Solid Edge part; units mm, degrees
sketch "Sketch1" plane through (0, 0, 0) normal (0, 0, 1) x (1, 0, 0)
  circle A0 centre (0, 0) radius 3.3
extrude "Protrusion1" add sketch "Sketch1" along normal blind 4.8
sketch "Sketch2" plane through (0, 0, 4.8) normal (0, 0, 1) x (1, 0, 0)
  circle A0 centre (0, 0) radius 2.25
extrude "nail_base" cut sketch "Sketch2" against normal blind 0.8
sketch "Sketch3" plane through (0, 0, 4) normal (0, 0, 1) x (1, 0, 0)
  circle A0 centre (0, 0) radius 1.4
extrude "Cutout1" cut sketch "Sketch3" against normal through all
sketch "Sketch4" plane through (0, 0, 0) normal (0, 0, -1) x (0, 1, 0)
  circle A0 centre (0, 0) radius 2.2
extrude "servo_mounting" cut sketch "Sketch4" against normal blind 2.8
sketch "Sketch5" plane through (0, 0, 2.4) normal (0, 0, -1) x (1, 0, 0)
  line L0 (-3.2891, 0.268) -> (-1.95, 16.7)
  arc A0 (-1.95, 16.7) -> (1.95, 16.7) centre (0, 16.1825) cw
  line L1 (3.2891, 0.268) -> (1.95, 16.7)
  arc A1 (-3.2891, 0.268) -> (3.2891, 0.268) centre (0, 0) cw
extrude "connector" add sketch "Sketch5" against normal blind 2
sketch "Sketch6" plane through (0, 0, 0) normal (0, 0, 1) x (1, 0, 0)
  circle A0 centre (0, -4.9) radius 0.6
  circle A1 centre (0, -6.8333) radius 0.6
  circle A2 centre (0, -8.7667) radius 0.6
  circle A3 centre (0, -10.7) radius 0.6
  circle A4 centre (0, -12.6333) radius 0.6
  circle A5 centre (0, -14.5667) radius 0.6
  circle A6 centre (0, -16.5) radius 0.6
extrude "Cutout2" cut sketch "Sketch6" along normal through all
The listing builds one solid part. Answer for the finished solid, in the listing's coordinates (mm). A direction names the side the tool comes from. Give positions to 0.01 mm unless a question says otherwise; leave off trailing zeros. Order: outer loops, then holes, each group sorted by start corner. A loop starts at its lowest first (then second) coordinate and runs counter-clockwise, first axis right, second up.
Item 1: The part is cut by section A-A, the plane y = 0. Give the vertices of the cut face in (x, z), and give its area (3 significant figures).
From the geometry:
outline: (-3.3, 0) - (-2.2, 0) - (-2.2, 2.8) - (-1.4, 2.8) - (-1.4, 4) - (-2.25, 4) - (-2.25, 4.8) - (-3.3, 4.8) - close; (1.4, 2.8) - (2.2, 2.8) - (2.2, 0) - (3.3, 0) - (3.3, 4.8) - (2.25, 4.8) - (2.25, 4) - (1.4, 4) - close
area: 12.4 mm2
Item 2: For a pull along X with two mould halves and no side action, classify faces 4 (the face through (1.4, -2.2, 4.8)), 5 (the face through (0.277, -14.034, 3.386)), 6 (the face through (-2.63, -8.37, 3.39)) as pulls with the +X half, pulls with the -X half, needs draft (parallel to the pull), parting line crosses it, or undercut.
From the geometry:
face 4: needs draft
face 5: undercut
face 6: pulls with the -X half
Item 3: The part is cut by section D-D, the plane y = -16.5. Give the vertices of the cut face in (x, z), and give its area (3 significant figures).
From the geometry:
outline: (-1.97, 2.4) - (-0.6, 2.4) - (-0.6, 4.4) - (-1.97, 4.4) - close; (0.6, 2.4) - (1.97, 2.4) - (1.97, 4.4) - (0.6, 4.4) - close
area: 5.47 mm2
Item 4: Which of the six approach directions +Z, -Z, +X, -X, +Y, -Y give full straight-line access (tool end or side, diameter ignored) to faces 1 (the face through (-0.078, -17.095, 3.386)), 2 (the face through (-0.29, 2.23, 4.41)), 3 (the face through (0.66, 2.1, 1.38))?
From the geometry:
face 1: +Z, -Z
face 2: +Z
face 3: -Z
Item 5: Find the intervals of material crossed by probe 1 along X at (y, z) = (-16.5, 3.8); probe 2 along Z at (x, y) = (1, -6); probe 3 along Y at (x, z) = (1, 1.25), in increasing order.
From the geometry:
probe 1: x = -1.97 to -0.6, 0.6 to 1.97
probe 2: z = 2.4 to 4.4
probe 3: y = -3.14 to -1.96, 1.96 to 3.14
Item 6: Given pin 1 Ø1.9 at (x, y) = (0, -6.83) entering from +Z; pin 2 Ø3 at (x, y) = (-2.5, -9.5) entering from -Z; pin 3 Ø1.3 at (x, y) = (0, 1) entering from +Z; pin 4 Ø3.5 at (x, y) = (-1, -0.5) entering from -Z, each flat-ended and moving along its own axis, determine where each tip first touches the part or whether it passes through.
From the geometry:
pin 1: stops at z = 4.4
pin 2: stops at z = 2.4
pin 3: stops at z = 4
pin 4: stops at z = 0
Item 7: The part is cut by section B-B, the plane x = -1. Give the vertices of the cut face in (y, z).
From the geometry:
outline: (-17.93, 2.4) - (-3.14, 2.4) - (-3.14, 0) - (-1.96, 0) - (-1.96, 2.8) - (-0.98, 2.8) - (-0.98, 4) - (-2.02, 4) - (-2.02, 4.8) - (-3.14, 4.8) - (-3.14, 4.4) - (-17.93, 4.4) - close; (0.98, 2.8) - (1.96, 2.8) - (1.96, 0) - (3.14, 0) - (3.14, 4.8) - (2.02, 4.8) - (2.02, 4) - (0.98, 4) - close
Item 8: The part is cut by section C-C, the plane z = 1.55. Give the vertices of the cut face in (x, y).
From the geometry:
outline: circle Ø6.6 at (0, 0); hole circle Ø4.4 at (0, 0)
